```python
from build123d import *

# Parameters (mm, degrees)
F0_R     = 15.5
F0_R_2   = 13.5
F1_DEPTH = 20
F2_W     = 5
F2_H     = 10.8510299228
F3_DEPTH = 10
F5_DEPTH = 25
F6_R     = 2.75
F7_DEPTH = 15


with BuildPart() as f1:
    # F0 (on Top) → F1 (new body)
    with BuildSketch(Plane.XY):
        with Locations((-43.3026812971, 10.8993155882)):
            Circle(F0_R)
        with Locations((-43.3026812971, 10.8993155882)):
            Circle(F0_R_2, mode=Mode.SUBTRACT)
    extrude(amount=F1_DEPTH)

    # F2 (on face) → F3 (join)
    with BuildSketch(Plane.XY.offset(20)):
        with Locations((-47.8026812971, 31.8248305496)):
            Rectangle(F2_W, F2_H)
        with Locations((-38.8026812971, 31.8248305496)):
            Rectangle(F2_W, F2_H)
        with BuildLine():
            Line((-50.3026812971, 24.7286322741), (-50.3026812971, 26.3993155882))
            Line((-50.3026812971, 26.3993155882), (-63.3026812971, 26.3993155882))
            Line((-63.3026812971, 26.3993155882), (-63.3026812971, 21.3993155882))
            Line((-63.3026812971, 21.3993155882), (-54.7044355481, 21.3993155882))
            ThreePointArc((-54.7044355481, 21.3993155882), (-52.6529340892, 23.2614664012), (-50.3026812971, 24.7286322741))
        make_face()
        with BuildLine():
            Line((-23.3026812971, 26.3993155882), (-36.3026812971, 26.3993155882))
            Line((-36.3026812971, 26.3993155882), (-36.3026812971, 24.7286322741))
            ThreePointArc((-36.3026812971, 24.7286322741), (-33.9524285049, 23.2614664012), (-31.9009270461, 21.3993155882))
            Line((-31.9009270461, 21.3993155882), (-23.3026812971, 21.3993155882))
            Line((-23.3026812971, 21.3993155882), (-23.3026812971, 26.3993155882))
        make_face()
        with BuildLine():
            Line((-45.3026812971, 26.2697417371), (-45.3026812971, 26.3993155882))
            Line((-45.3026812971, 26.3993155882), (-50.3026812971, 26.3993155882))
            Line((-50.3026812971, 26.3993155882), (-50.3026812971, 24.7286322741))
            ThreePointArc((-50.3026812971, 24.7286322741), (-47.8681773921, 25.711683576), (-45.3026812971, 26.2697417371))
        make_face()
        with BuildLine():
            Line((-36.3026812971, 26.3993155882), (-41.3026812971, 26.3993155882))
            Line((-41.3026812971, 26.3993155882), (-41.3026812971, 26.2697417371))
            ThreePointArc((-41.3026812971, 26.2697417371), (-38.737185202, 25.711683576), (-36.3026812971, 24.7286322741))
            Line((-36.3026812971, 24.7286322741), (-36.3026812971, 26.3993155882))
        make_face()
        with BuildLine():
            ThreePointArc((-43.3026812971, -4.6006844118), (-49.5276310961, -3.2957539784), (-54.7044355481, 0.3993155882))
            Line((-54.7044355481, 0.3993155882), (-65.8026812971, 0.3993155882))
            Line((-65.8026812971, 0.3993155882), (-65.8026812971, -4.6006844118))
            Line((-65.8026812971, -4.6006844118), (-43.3026812971, -4.6006844118))
        make_face()
        with BuildLine():
            ThreePointArc((-31.9009270461, 0.3993155882), (-37.0777314981, -3.2957539784), (-43.3026812971, -4.6006844118))
            Line((-43.3026812971, -4.6006844118), (-20.8026812971, -4.6006844118))
            Line((-20.8026812971, -4.6006844118), (-20.8026812971, 0.3993155882))
            Line((-20.8026812971, 0.3993155882), (-31.9009270461, 0.3993155882))
        make_face()
    extrude(amount=-F3_DEPTH)

    # F4 (on face) → F5 (cut)
    with BuildSketch(Plane.XY.offset(20)):
        with BuildLine():
            Line((-41.3026812971, 27.4977236986), (-45.3026812971, 27.4977236986))
            Line((-45.3026812971, 27.4977236986), (-45.3026812971, 26.2697417371))
            ThreePointArc((-45.3026812971, 26.2697417371), (-43.3026812971, 26.3993155882), (-41.3026812971, 26.2697417371))
            Line((-41.3026812971, 26.2697417371), (-41.3026812971, 27.4977236986))
        make_face()
        with BuildLine():
            ThreePointArc((-41.3026812971, 26.2697417371), (-43.3026812971, 26.3993155882), (-45.3026812971, 26.2697417371))
            Line((-45.3026812971, 26.2697417371), (-45.3026812971, 24.250345511))
            ThreePointArc((-45.3026812971, 24.250345511), (-43.3026812971, 24.3993155882), (-41.3026812971, 24.250345511))
            Line((-41.3026812971, 24.250345511), (-41.3026812971, 26.2697417371))
        make_face()
    extrude(amount=-F5_DEPTH, mode=Mode.SUBTRACT)

    # F6 (on face) → F7 (cut)
    with BuildSketch(Plane(origin=(-50.3026812971, 0, 0), x_dir=(0, -1, 0), z_dir=(-1, 0, 0))):
        with Locations((-32.500345511, 14.75)):
            Circle(F6_R)
    extrude(amount=-F7_DEPTH, mode=Mode.SUBTRACT)


solid = f1.part
```
Build history of the part. All positions in model axes, mm. A direction names the side the tool comes from. Give positions to 0.01 mm unless a question says otherwise; leave off trailing zeros. Loops run counter-clockwise (first coordinate to the right, second up) from the corner with the lowest first, then second, coordinate; pieces in that order, holes last. Notation, with made-up numbers: (31.25, 18) - (73.25, 18) arc R24 cw to (73.25, 49) - close; hole circle Ø9 at (49.5, 36). An arc over 180 degrees is marked (long way). Use a Markdown table: item, result.
(1) Band-saw the part on A-A (y = 28.5). Give the cut face in (x, z), and give its area (3 significant figures).
Taken from the geometry:
| item | result |
|---|---|
| outline | (-50.3, 10) - (-45.3, 10) - (-45.3, 20) - (-50.3, 20) - close; (-41.3, 10) - (-36.3, 10) - (-36.3, 20) - (-41.3, 20) - close |
| area | 100 mm2 |
(2) Which spindle directions (+Z, -Z, +X, -X, +Y, -Y) get a long thin tool onto all of the face, cutting with end or side? Do faces 1 (the face through (-60, 0.399, 15)), 2 (the face through (-41.303, 29, 15)), 3 (the face through (-57, -2, 10)), 4 (the face through (-50.303, 29, 15)), 5 (the face through (-30, 26.399, 15)). Say none if no direction does.
Taken from the geometry:
| item | result |
|---|---|
| face 1 | +Z, -Z, -X |
| face 2 | +Z, -Z, +Y |
| face 3 | -Z, -X, -Y |
| face 4 | +Z, -Z, -X, +Y |
| face 5 | +Z, -Z, +X, +Y |
(3) Band-saw the part on C-C (x = -39.5). Give the cut face in (y, z), and give its area (3 significant figures).
Taken from the geometry:
| item | result |
|---|---|
| outline | (-4.6, 10) - (-4.13, 10) - (-4.13, 0) - (-2.05, 0) - (-2.05, 20) - (-4.6, 20) - close; (23.85, 0) - (25.93, 0) - (25.93, 10) - (37.25, 10) - (37.25, 20) - (23.85, 20) - close; hole circle Ø5.5 at (32.5, 14.75) |
| area | 177 mm2 |
(4) Drop flat-ended pins along their axis: pin 1 Ø8 at (x, y) = (-31.5, 26.5) entering from -Z; pin 2 Ø12 at (y, z) = (11, 10.5) entering from -X; pin 3 Ø4 at (x, z) = (-33, 3.5) entering from +Y; pin 4 Ø4.5 at (y, z) = (32.5, 14.75) entering from +X. Give the stop position or say it passes through.
Taken from the geometry:
| item | result |
|---|---|
| pin 1 | z = 10 |
| pin 2 | x = -58.8 |
| pin 3 | y = 23.99 |
| pin 4 | through |
(5) Band-saw the part on D-D (y = 13). Give the cut face in (x, z).
Taken from the geometry:
| item | result |
|---|---|
| outline | (-58.66, 0) - (-56.64, 0) - (-56.64, 20) - (-58.66, 20) - close; (-29.97, 0) - (-27.95, 0) - (-27.95, 20) - (-29.97, 20) - close |
(6) Band-saw the part on B-B (z = 14.75). Give the cut face in (x, y), and give its area (3 significant figures).
Taken from the geometry:
| item | result |
|---|---|
| outline | (-65.8, -4.6) - (-20.8, -4.6) - (-20.8, 0.4) - (-31.9, 0.4) arc R15.5 ccw to (-31.9, 21.4) - (-23.3, 21.4) - (-23.3, 26.4) - (-36.3, 26.4) - (-36.3, 29.75) - (-41.3, 29.75) - (-41.3, 24.25) arc R13.5 cw (long way) to (-45.3, 24.25) - (-45.3, 29.75) - (-50.3, 29.75) - (-50.3, 26.4) - (-63.3, 26.4) - (-63.3, 21.4) - (-54.7, 21.4) arc R15.5 ccw to (-54.7, 0.4) - (-65.8, 0.4) - close; (-50.3, 35.25) - (-45.3, 35.25) - (-45.3, 37.25) - (-50.3, 37.25) - close; (-41.3, 35.25) - (-36.3, 35.25) - (-36.3, 37.25) - (-41.3, 37.25) - close |
| area | 495 mm2 |
(7) Wall check: line 1 along X through (y, z) = (26, 13); line 2 along X through (y, z) = (28.5, 14.75); line 3 along Z through (x, y) = (-30, 23). Give the ranges that are in metal, low to high.
Taken from the geometry:
| item | result |
|---|---|
| line 1 | -63.3 to -45.3, -41.3 to -23.3 |
| line 2 | -50.3 to -45.3, -41.3 to -36.3 |
| line 3 | 10 to 20 |
(8) Pull direction Z, two halves, no side cores. Call faces 6 (the face through (-63.303, 24, 15)), 7 (the face through (-47.838, 35.248, 14.871)), 8 (the face through (-45, -3, 0)): +Z half, -Z half, draft (parallel to the pull), parting line (faces both ways), or undercut.
Taken from the geometry:
| item | result |
|---|---|
| face 6 | draft |
| face 7 | undercut |
| face 8 | -Z half |
